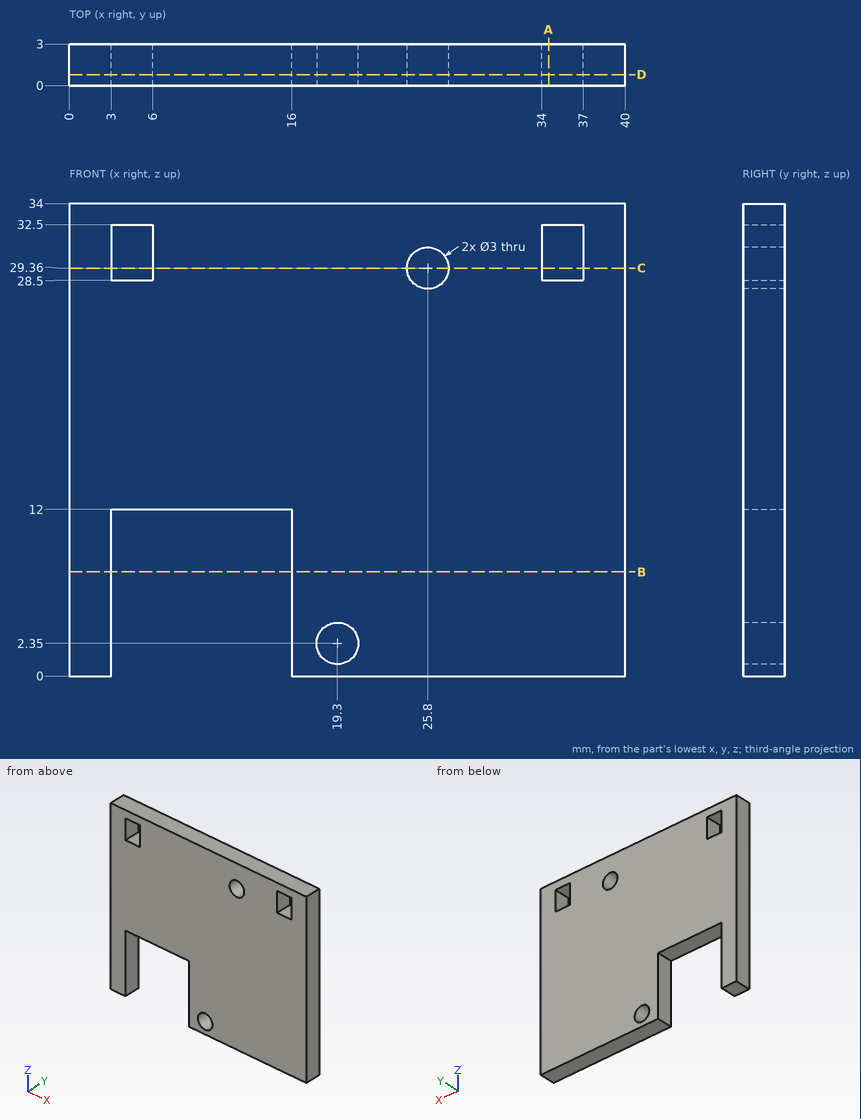
Source: three-view drawing plus pictorial views. Frame: mm from the lowest corner of the part. Round coordinates to 2 decimals unless told otherwise and drop trailing zeros. Order: outer loops, then holes, each group sorted by start corner. A loop starts at its lowest first (then second) coordinate and runs counter-clockwise, first axis right, second up. Notation, with made-up numbers: (30, 49.5) -> (35, 49.5) arc R18 cw to (35, 82.5) -> close; hole circle Ø6 at (31, 34). An arc over 180 degrees is marked (long way). Use CSV: the item, a comma, the result in double quotes. Start each with the question number.
1) Section D-D (y = 0.8). Return the cut outline in (x, z), and give its area (3 significant figures).
2) Section C-C (z = 29.36). Return the cut outline in (x, y).
3) Section A-A (x = 34.5). Return the cut outline in (y, z).
4) Section B-B (z = 7.5). Return the cut outline in (x, y).
5) Material intervals for line 1 along X through (y, z) = (1.8, 29.36); line 2 along Z through (x, y) = (4, 0.3); line 3 along Z through (x, y) = (19.3, 0.9), sorted ascending. Write a range as from..to.
6) First-contact query: pin 1 Ø1.5 at (x, y) = (5, 1.5) entering from -Z. Flat tip, straight axial feed; report the tip coordinate or a pass-through.
Returned:
1,outline,"(0, 0) -> (3, 0) -> (3, 12) -> (16, 12) -> (16, 0) -> (40, 0) -> (40, 34) -> (0, 34) -> close; hole (3, 28.5) -> (6, 28.5) -> (6, 32.5) -> (3, 32.5) -> close; hole circle Ø3 at (19.3, 2.35); hole circle Ø3 at (25.8, 29.36); hole (34, 28.5) -> (37, 28.5) -> (37, 32.5) -> (34, 32.5) -> close"
1,area,"1,170 mm²"
2,outline,"(0, 0) -> (3, 0) -> (3, 3) -> (0, 3) -> close; (6, 0) -> (24.3, 0) -> (24.3, 3) -> (6, 3) -> close; (27.3, 0) -> (34, 0) -> (34, 3) -> (27.3, 3) -> close; (37, 0) -> (40, 0) -> (40, 3) -> (37, 3) -> close"
3,outline,"(0, 0) -> (3, 0) -> (3, 28.5) -> (0, 28.5) -> close; (0, 32.5) -> (3, 32.5) -> (3, 34) -> (0, 34) -> close"
4,outline,"(0, 0) -> (3, 0) -> (3, 3) -> (0, 3) -> close; (16, 0) -> (40, 0) -> (40, 3) -> (16, 3) -> close"
5,line 1,"x = 0..3, 6..24.3, 27.3..34, 37..40"
5,line 2,"z = 12..28.5, 32.5..34"
5,line 3,"z = 0..0.85, 3.85..34"
6,pin 1,"stops at z = 12"
